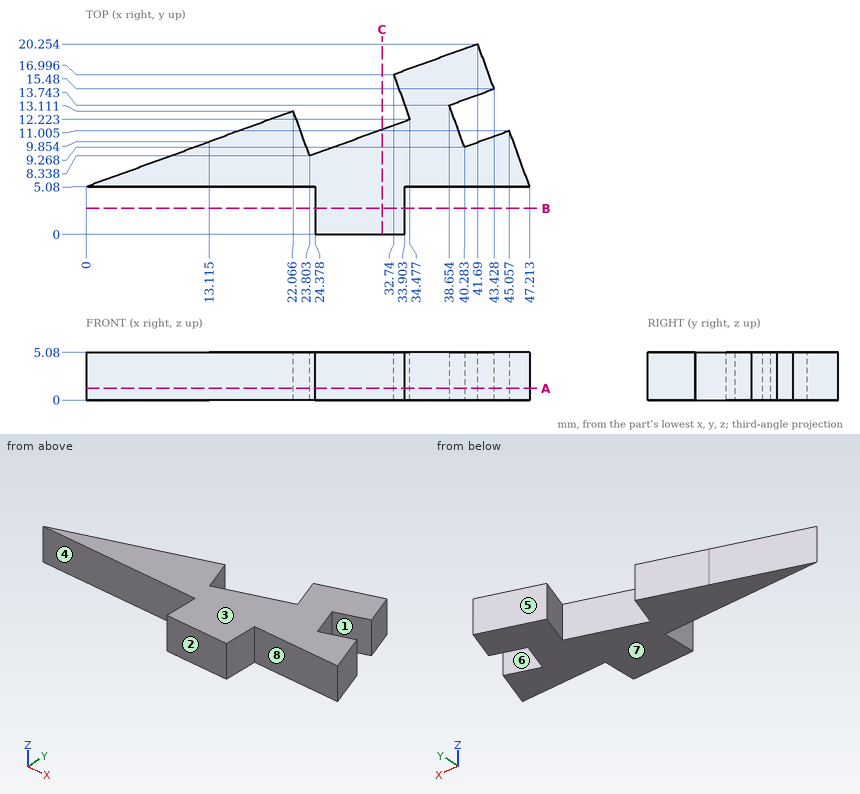
For this review, use the dimensioned drawing (mm, ordinates from the lowest corner) and the shaded views. A direction names the side the tool comes from. Give positions to 0.01 mm unless a question says otherwise; leave off trailing zeros. Loops run counter-clockwise (first coordinate to the right, second up) from the corner with the lowest first, then second, coordinate; pieces in that order, holes last.
Item 1: Insertion check: pin 1 (2.5 mm diameter, centred on y = 1.5, z = 2, fed in from -X); pin 2 (1.5 mm diameter, centred on y = 11.5, z = 4.5, fed in from +X); pin 3 (2.5 mm diameter, centred on y = 2, z = 3.5, fed in from +X). Each pin has a flat end and moves straight along its axis. Give the tip position at first contact, or say it passes through.
Item 2: Take a section at A-A, the plane z = 1.25. State the section outline as (x, y) points (1 decimal).
Item 3: Draft analysis for pull direction Y (two halves, no side actions). For the marked faces 1, 2 and 3, state which applies: +Y half, -Y half, draft (parallel to the pull), parting line (faces both ways), or undercut.
Item 4: Take a section at B-B, the plane y = 2.75. State the section outline as (x, z) points.
Item 5: For line 1 along X through (y, z) = (3, 2.55); line 2 along Y through (x, z) = (41, 4.6); line 3 along Y through (x, z) = (27.5, 1.15), list the stretches that pass through material, from the lowest coordinate up.
Item 6: Take a section at C-C, the plane x = 31.5. State the section outline as (y, z) points, and give its area (3 significant figures).
Item 7: Tool access review of the marked faces 4, 5, 6, 7 and 8: name each direction out of +Z, -Z, +X, -X, +Y, -Y from which nothing blocks a thin tool from reaching the whole face with its end or side.
Calculated:
1. pin 1: stops at x = 24.38
1. pin 2: stops at x = 45.15
1. pin 3: stops at x = 33.9
2. outline: (0, 5.1) - (24.4, 5.1) - (24.4, 0) - (33.9, 0) - (33.9, 5.1) - (47.2, 5.1) - (45.1, 11) - (40.3, 9.3) - (38.7, 13.7) - (43.4, 15.5) - (41.7, 20.3) - (32.7, 17) - (34.5, 12.2) - (23.8, 8.3) - (22.1, 13.1) - close
3. face 1: undercut
3. face 2: -Y half
3. face 3: draft
4. outline: (24.38, 0) - (33.9, 0) - (33.9, 5.08) - (24.38, 5.08) - close
5. line 1: x = 24.38 to 33.9
5. line 2: y = 5.08 to 9.53, 14.6 to 20
5. line 3: y = 0 to 9.68
6. outline: (0, 0) - (11.14, 0) - (11.14, 5.08) - (0, 5.08) - close
6. area: 56.6 mm2
7. face 4: +Z, -Z, -X, -Y
7. face 5: +Z, -Z, -X, +Y
7. face 6: +Z, -Z
7. face 7: -Z, +X, -X, +Y, -Y
7. face 8: +Z, -Z, +X, -Y
